Autodesk Fusion 360 part; units mm, degrees
sketch "スケッチ3" plane through (0, 0, 0) normal (0, 1, 0) x (1, 0, 0)
  line L0 (0, 0) -> (24.15, 0)
  line L1 (24.15, 0) -> (24.15, -67.65)
  line L2 (24.15, -67.65) -> (0, -67.65)
  line L3 (0, -67.65) -> (0, 0)
  arc A0 (21.15, 0) -> (23.7006, 1.2675) centre (21.15, 3.2) ccw
  line L4 (21.15, 3.2) -> (21.15, 0) construction
  line L5 (21.15, 3.2) -> (23.7006, 1.2675) construction
  line L6 (24.15, 0) -> (24.15, 1.12)
  arc A1 (24.15, 1.12) -> (23.7006, 1.2675) centre (23.9011, 1.12) ccw
  line L7 (22.5, -67.65) -> (22.5, 0.2987)
  line L8 (0, -66) -> (24, -66)
  circle A2 centre (19.575, -10) radius 1.5
  line L9 (12.075, -67.65) -> (12.075, 0)
  circle A3 centre (19.575, -62.5) radius 1.5
  arc A4 (0.4494, 1.2675) -> (3, 0) centre (3, 3.2) ccw
  line L10 (0, 0) -> (0, 1.12)
  arc A5 (0.4494, 1.2675) -> (0, 1.12) centre (0.2489, 1.12) ccw
  line L11 (1.65, -67.65) -> (1.65, 0.2987)
  circle A6 centre (4.575, -62.5) radius 1.5
  circle A7 centre (4.575, -10) radius 1.5
  circle A8 centre (6.575, -46.5) radius 1
  circle A9 centre (19.575, -62.5) radius 4.5
  circle A10 centre (19.575, -10) radius 4.5
  circle A11 centre (4.575, -62.5) radius 4.5
  circle A12 centre (4.575, -10) radius 4.5
  point P0 (21.15, 0)
  point P1 (21.15, 3.2)
  point P2 (23.9, 0.8469)
  dimension "d1" = 24.15
  dimension "d4" = 3.2
  dimension "d5" = 3
  dimension "d6" = 52.85
  dimension "d10" = 1.12
  dimension "d12" = 1.65
  dimension "d13" = 1.65
  dimension "d14" = 3
  dimension "d15" = 10
  dimension "d16" = 12.075
  dimension "d17" = 7.5
  dimension "d18" = 3
  dimension "d19" = 62.5
  dimension "d20" = 66
  dimension "d21" = 2
  dimension "d22" = 5.5
  dimension "d23" = 46.5
  dimension "d31" = 9
  dimension "d32" = 9
  dimension "d33" = 7.5
extrude "押し出し1" add sketch "スケッチ3" along normal blind 13.35 contours L0 L8 L9 L11 A11 A12 | L0 A4 L11 | L0 L7 L8 L9 A9 A10 | L0 L3 L8 L11 A11 A12 | L0 A4 L10 A5 L11 | L0 A0 L7 | L2 L8 L9 L11 A11 | L2 L7 L8 L9 A9 | L11 A12 | L11 A12 | L0 A0 L6 A1 L7 | L0 L1 L2 L7 A9 A10 | L8 A11 | L8 L11 A11 | L7 L8 A9 | L8 A9 | L2 L3 L8 L11 | L7 A10 | L7 A10 | L8 L11 A11 | L7 L8 A9 | L7 A9 | L11 A11 | A2 | A3 | A6 | A7 | A8
extrude "押し出し3" cut sketch "スケッチ3" against normal blind 11.7 from surface at 13.35 contours L0 L8 L9 L11 A11 A12 | L0 A4 L11 | L0 L7 L8 L9 A9 A10 | L0 A0 L7 | L11 A12 | L8 L11 A11 | L7 L8 A9 | L7 A10 | L8 L11 A11 | L7 L8 A9 | A2 | A3 | A6 | A7 | A8 picked at (2.125, -10) picked at (22.025, -10)
extrude "押し出し4" add sketch "スケッチ3" along normal blind 9.25 contours L11 A12 | L8 A11 | L8 L11 A11 | L7 L8 A9 | L8 A9 | L7 A10 picked at (2.125, -10) picked at (4.6124, -65.3319) picked at (19.5376, -65.3319) picked at (22.025, -10)
extrude "押し出し5" add sketch "スケッチ3" along normal blind 2.75 contours A2 | A3 | A6 | A7
Build history of the part. All positions in model axes, mm. A direction names the side the tool comes from. Round coordinates to 2 decimals unless told otherwise and drop trailing zeros. Loops run counter-clockwise (first coordinate to the right, second up) from the corner with the lowest first, then second, coordinate; pieces in that order, holes last. Notation, with made-up numbers: (74.25, 32.25) -> (131.25, 32.25) arc R21 ccw to (131.25, 49.25) -> close; hole circle Ø2 at (26.5, 12.5). An arc over 180 degrees is marked (long way). Answer in a Markdown table with one row per item.
Item 1: Saw through at D-D (z = 62.5). Write the cut outline in (x, y) (3 decimals).
Answers below:
| item | result |
|---|---|
| outline | (0, 0) -> (24.15, 0) -> (24.15, 13.35) -> (22.5, 13.35) -> (22.5, 9.25) -> (21.075, 9.25) -> (21.075, 2.75) -> (18.075, 2.75) -> (18.075, 9.25) -> (15.075, 9.25) -> (15.075, 1.65) -> (9.075, 1.65) -> (9.075, 9.25) -> (6.075, 9.25) -> (6.075, 2.75) -> (3.075, 2.75) -> (3.075, 9.25) -> (1.65, 9.25) -> (1.65, 13.35) -> (0, 13.35) -> close |
Item 2: Saw through at A-A (z = 17.5). Write the cut outline in (x, y), and give its area (3 significant figures).
Answers below:
| item | result |
|---|---|
| outline | (0, 0) -> (24.15, 0) -> (24.15, 13.35) -> (22.5, 13.35) -> (22.5, 1.65) -> (1.65, 1.65) -> (1.65, 13.35) -> (0, 13.35) -> close |
| area | 78.5 mm² |
Item 3: Pin check, flat tips, straight feed: pin 1 (2 mm diameter, centred on x = 10.5, y = 10, fed in from -Z); pin 2 (2.5 mm diameter, centred on x = 19, z = 10.5, fed in from +Y); pin 3 (3.5 mm diameter, centred on x = 4.575, z = 62.5, fed in from -Y); pin 4 (0.8 mm diameter, centred on x = 8, y = 1, fed in from -Z). Stop position of each tip, or through.
Answers below:
| item | result |
|---|---|
| pin 1 | stops at z = 66 |
| pin 2 | stops at y = 9.25 |
| pin 3 | stops at y = 0 |
| pin 4 | stops at z = 0 |
Item 4: Which spindle directions (+Z, -Z, +X, -X, +Y, -Y) get a long thin tool onto all of the face, cutting with end or side? Do faces 1 (the cylindrical face through (23.144, 6.582, -0.697)), 2 (the flat face through (17.9, 9.25, 9.9)), 3 (the flat face through (12, 0, 33)), 4 (the flat face through (20, 2.75, 62)). Say none if no direction does.
Answers below:
| item | result |
|---|---|
| face 1 | -Z, +Y, -Y |
| face 2 | -Z, +Y |
| face 3 | +Z, -Z, +X, -X, -Y |
| face 4 | +Y |
Item 5: Drill centre lines: L1, parallel to X at y = 6.25, z = 62.5 (3 decimals); L2, parallel to X at y = 4.25, z = 42; L3, parallel to Y at x = 12.75, z = 54. Where is each one in solid material? Low to high. Write a range as [from, to].
Answers below:
| item | result |
|---|---|
| L1 | x = [0, 3.075], [6.075, 9.075], [15.075, 18.075], [21.075, 24.15] |
| L2 | x = [0, 1.65], [22.5, 24.15] |
| L3 | y = [0, 1.65] |
Item 6: Saw through at C-C (x = 12.25). Write the cut outline in (y, z), and give its area (3 significant figures).
Answers below:
| item | result |
|---|---|
| outline | (0, 0) -> (1.65, 0) -> (1.65, 66) -> (13.35, 66) -> (13.35, 67.65) -> (0, 67.65) -> close |
| area | 131 mm² |
Item 7: Mould opens along Z. For faces 5 (the cylindrical face through (19.25, 5.954, 8.536)), 6 (the flat face through (6, 9.25, 11)), 7 (the flat face through (12, 1, 0)) say: +Z half, -Z half, draft (parallel to the pull), parting line (faces both ways), or undercut.
Answers below:
| item | result |
|---|---|
| face 5 | undercut |
| face 6 | draft |
| face 7 | -Z half |
Item 8: Saw through at B-B (y = 10). Write the cut outline in (x, z).
Answers below:
| item | result |
|---|---|
| outline | (0, -1.12) arc R0.25 ccw to (0.45, -1.27) arc R3.2 cw to (1.65, -0.3) -> (1.65, 66) -> (22.5, 66) -> (22.5, -0.3) arc R3.2 cw to (23.7, -1.27) arc R0.25 ccw to (24.15, -1.12) -> (24.15, 67.65) -> (0, 67.65) -> close |
